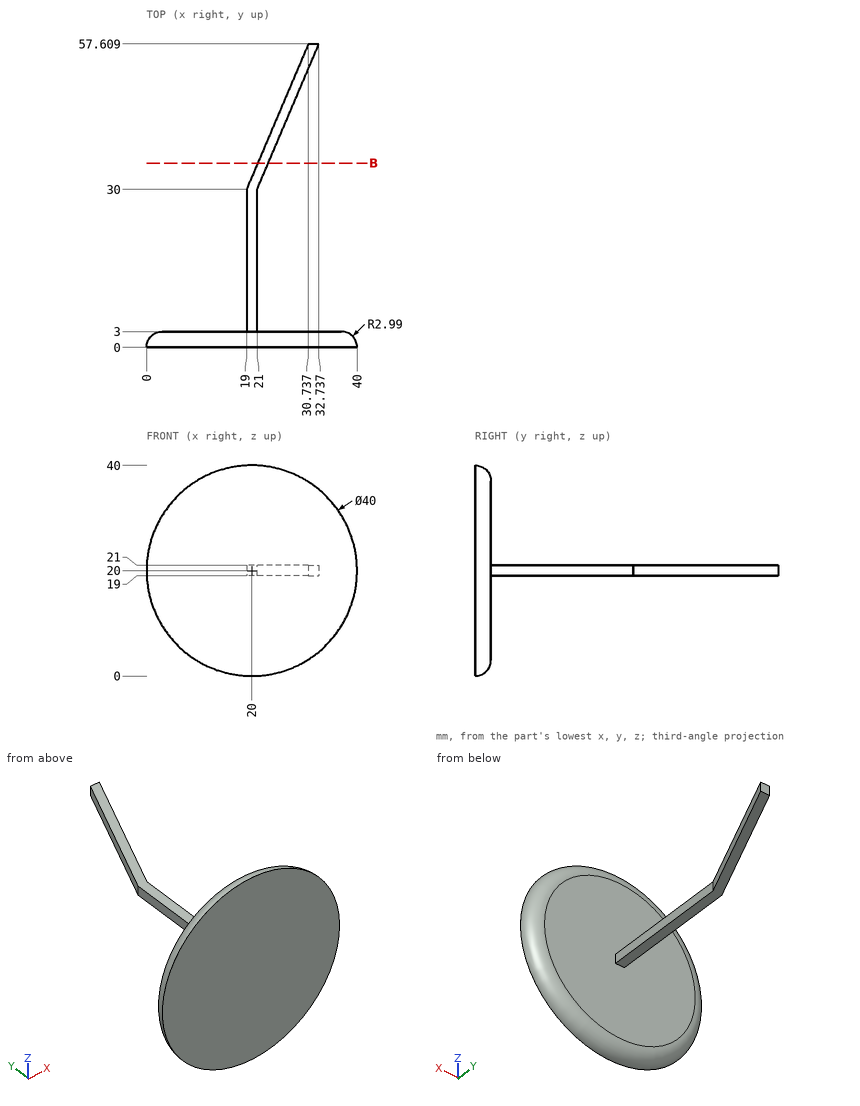
Check sheet for the drawn part. Datum: minimum x, y, z corner. Units: mm. Give positions to 0.01 mm unless a question says otherwise; leave off trailing zeros. Write each loop counter-clockwise with the first axis right and the second up, starting at its lowest first coordinate (ties: lowest second). Pieces come first, ordered by that corner, then holes.
(1) Gauge pin test, flat ends, axial feed: pin 1 (2 mm diameter, centred on x = 30, z = 14, fed in from +Y); pin 2 (1 mm diameter, centred on y = 10.5, z = 20, fed in from -X); pin 3 (7 mm diameter, centred on x = 27.5, y = 33.5, fed in from +Z); pin 4 (0.6 mm diameter, centred on y = 21, z = 20, fed in from +X). Record the tip position at first contact, or that the pin passes through.
(2) Material ranges on line 1 (Y direction, x = 17.5, z = 33); line 2 (Y direction, x = 29, z = 4.5), recorded low to high.
(3) Cross-section at B-B (y = 35). Enter the section's corners in (x, z) (1 decimal).
Worked out:
1. pin 1: stops at y = 3
1. pin 2: stops at x = 19
1. pin 3: passes through
1. pin 4: stops at x = 21
2. line 1: y = 0 to 3
2. line 2: y = 0 to 2.86
3. outline: (21.1, 19) - (23.1, 19) - (23.1, 21) - (21.1, 21) - close
